from build123d import *

# Parameters (mm, degrees)
CUT_EXTRUDE_12_DEPTH      = 102.948516419
CUT_EXTRUDE_12_DEPTH_BACK = 102.948516419
CUT_EXTRUDE_START         = 61
CUT_EXTRUDE_5_R0_25_DEPTH = 31


with BuildPart() as part:
    # Эскиз1 → Revolve 289 (revolve)
    with BuildSketch(Plane.XY, mode=Mode.PRIVATE) as revolve_289_sk:
        with BuildLine():
            Line((0, 32.5), (37, 32.5))
            Line((37, 32.5), (64.745695, 25.068113))
            ThreePointArc((64.745695, 25.068113), (65.002224223, 25.017098236), (65.263217049, 24.999995817))
            Line((65.263217049, 24.999995817), (69.749999449, 24.999995817))
            Line((69.749999449, 24.999995817), (70.749999449, 23.999995817))
            Line((70.749999449, 23.999995817), (70.749999449, 19.499995817))
            Line((70.749999449, 19.499995817), (79.25, 19.499995817))
            Line((79.25, 19.499995817), (79.25, 24))
            Line((79.25, 24), (80.25, 25))
            Line((80.25, 25), (88, 25))
            Line((88, 25), (91, 22))
            Line((91, 22), (91, 11))
            Line((91, 11), (90, 10))
            Line((90, 10), (61, 10))
            Line((61, 10), (61, 19))
            ThreePointArc((61, 19), (60.707106781, 19.707106781), (60, 20))
            Line((60, 20), (25, 20))
            Line((25, 20), (25, 27.1))
            ThreePointArc((25, 27.1), (24.882842712, 27.382842712), (24.6, 27.5))
            Line((24.6, 27.5), (0, 27.5))
            Line((0, 27.5), (0, 32.5))
        make_face()
    revolve(revolve_289_sk.sketch.rotate(Axis((0, 0, 0), (1, 0, 0)), 90), axis=Axis((0, 0, 0), (1, 0, 0)))

    # Эскиз2 → Наклон торца 12 градусов (cut, two sides: drawn at the far end of the back side and taken through both)
    with BuildSketch(Plane(origin=(0, 0, 0), x_dir=(1, 0, 0), z_dir=(0, 1, 0)).offset(-CUT_EXTRUDE_12_DEPTH_BACK)):
        Polygon((-25, 50), (15.30407244, 50), (-5.951583727, -50), (-25, -50), align=None)
    extrude(amount=CUT_EXTRUDE_12_DEPTH + CUT_EXTRUDE_12_DEPTH_BACK, mode=Mode.SUBTRACT)

    # Эскиз3 → Паз 5 R0.25 (cut)
    with BuildSketch(Plane(origin=(0, 0, 0), x_dir=(0, 0, -1), z_dir=(1, 0, 0)).offset(CUT_EXTRUDE_START)):
        with BuildLine():
            Line((0, -2.5), (0, 2.5))
            Line((0, 2.5), (-12.05, 2.5))
            ThreePointArc((-12.05, 2.5), (-12.226776695, 2.426776695), (-12.3, 2.25))
            Line((-12.3, 2.25), (-12.3, -2.25))
            ThreePointArc((-12.3, -2.25), (-12.226776695, -2.426776695), (-12.05, -2.5))
            Line((-12.05, -2.5), (0, -2.5))
        make_face()
    extrude(amount=CUT_EXTRUDE_5_R0_25_DEPTH, mode=Mode.SUBTRACT)

    # Эскиз4 → Cut-Revolve M4 30 -1 (revolve, cut)
    with BuildSketch(Plane(origin=(0, 0, 0), x_dir=(1, 0, 0), z_dir=(0, -0.49999999999999994, 0.8660254037844387)), mode=Mode.PRIVATE) as cut_revolve_m4_30_1_sk:
        Polygon((17, -26), (18.7, -26), (18.7, -29.5), (20.5, -29.5), (20.5, -40), (17, -40), align=None)
    revolve(cut_revolve_m4_30_1_sk.sketch.rotate(Axis((17, -17.320508076, -10), (0, -0.8660254037844387, -0.49999999999999994)), 90), axis=Axis((17, -17.320508076, -10), (0, -0.8660254037844387, -0.49999999999999994)), mode=Mode.SUBTRACT)

    # Эскиз5 → Cut-Revolve M4 30 1 2 (revolve, cut)
    with BuildSketch(Plane(origin=(0, 0, 0), x_dir=(1, 0, 0), z_dir=(0, -0.49999999999999994, 0.8660254037844387)), mode=Mode.PRIVATE) as cut_revolve_m4_30_1_2_sk:
        Polygon((17, 26), (18.7, 26), (18.7, 29.5), (20.5, 29.5), (20.5, 40), (17, 40), align=None)
    revolve(cut_revolve_m4_30_1_2_sk.sketch.rotate(Axis((17, 17.320508076, 10), (0, 0.8660254037844387, 0.49999999999999994)), 90), axis=Axis((17, 17.320508076, 10), (0, 0.8660254037844387, 0.49999999999999994)), mode=Mode.SUBTRACT)

    # Эскиз6 → Cut-Revolve M4 150 -1 (revolve, cut)
    with BuildSketch(Plane(origin=(0, 0, 0), x_dir=(1, 0, 0), z_dir=(0, -0.49999999999999994, -0.8660254037844387)), mode=Mode.PRIVATE) as cut_revolve_m4_150_1_sk:
        Polygon((17, -26), (18.7, -26), (18.7, -29.5), (20.5, -29.5), (20.5, -40), (17, -40), align=None)
    revolve(cut_revolve_m4_150_1_sk.sketch.rotate(Axis((17, 17.320508076, -10), (0, 0.8660254037844387, -0.49999999999999994)), 90), axis=Axis((17, 17.320508076, -10), (0, 0.8660254037844387, -0.49999999999999994)), mode=Mode.SUBTRACT)

    # Эскиз7 → Cut-Revolve M4 150 1 2 (revolve, cut)
    with BuildSketch(Plane(origin=(0, 0, 0), x_dir=(1, 0, 0), z_dir=(0, -0.49999999999999994, -0.8660254037844387)), mode=Mode.PRIVATE) as cut_revolve_m4_150_1_2_sk:
        Polygon((17, 26), (18.7, 26), (18.7, 29.5), (20.5, 29.5), (20.5, 40), (17, 40), align=None)
    revolve(cut_revolve_m4_150_1_2_sk.sketch.rotate(Axis((17, -17.320508076, 10), (0, -0.8660254037844387, 0.49999999999999994)), 90), axis=Axis((17, -17.320508076, 10), (0, -0.8660254037844387, 0.49999999999999994)), mode=Mode.SUBTRACT)

    # Эскиз8 → Радиальное отверстие 3.6 цековка 7 (revolve, cut)
    with BuildSketch(Plane(origin=(0, 0, 0), x_dir=(1, 0, 0), z_dir=(0, 1, 0)), mode=Mode.PRIVATE) as cut_revolve_3_6_7_sk:
        Polygon((78, -8), (79.8, -8), (79.8, -15), (81.5, -15), (81.5, -35), (78, -35), align=None)
    revolve(cut_revolve_3_6_7_sk.sketch.rotate(Axis((78, 0, 0), (0, 0, 1)), 180), axis=Axis((78, 0, 0), (0, 0, 1)), mode=Mode.SUBTRACT)


solid = part.part
Geometry: final body of the model. Coordinates: model frame, mm. A direction names the side the tool comes from. Round coordinates to 2 decimals unless told otherwise and drop trailing zeros. Loops run counter-clockwise (first coordinate to the right, second up) from the corner with the lowest first, then second, coordinate; pieces in that order, holes last. Notation, with made-up numbers: M -29,-11 L 25,-11 A30 ccw 25,13 Z; hole C -24,24 d7. An arc over 180 degrees is marked long. One line per question, with ' | ' between items.
(1) Cut plane C-C on x = 49. Return the cut outline in (y, z), plus the area to 3 significant figures.
Check result:
outline: C 0,0 d58.57; hole C 0,0 d40 | area: 1,440 mm2
(2) Cut plane A-A on x = 72.5. Return the cut outline in (y, z).
Check result:
outline: C 0,0 d39; hole M -2.5,9.68 A10 ccw long 2.5,9.68 L 2.5,12.05 A0.25 ccw 2.25,12.3 L -2.25,12.3 A0.25 ccw -2.5,12.05 Z
(3) Contact query for flat-ended pins moving along their axis: P1, Ø8, axis at y = -12, z = -13, coming from the -X side; P2, Ø0.7, axis at x = 80.5, z = 11, coming from the +Y side; P3, Ø1.2, axis at x = 70.5, z = 11, coming from the -Y side; P4, Ø16, axis at y = 0, z = 0, coming from the +X side. Output: stop coordinate, or through.
Check result:
P1: stops at x = 25 | P2: stops at y = 22.62 | P3: stops at y = -22.34 | P4: passes through
(4) Cut plane B-B on y = 0. Give the number of separate pieces and of enclosed holes in the cut face, plus the area to 3 significant figures.
Check result:
separate pieces: 3 | enclosed holes: 0 | area: 1,620 mm2
(5) Access query for faces 5 (the cylindrical face through (67.538, 24.406, -5.42)), 6 (the cylindrical face through (42.26, -0.88, -19.98)), 7 (the cylindrical face through (81.497, -0.154, 18.959)). Directions: +Z, -Z, +X, -X, +Y, -Y. A direction counts if a zero-diameter tool reaches every point of the face in a straight line with its end or side. Return the directions, or none.
Check result:
face 5: +X | face 6: -X | face 7: +Z
(6) Material intervals for line 1 along X through (y, z) = (-16.5, 13); line 2 along Y through (x, z) = (69, 0); line 3 along X through (y, z) = (13, 19), sorted ascending. Write a range as from..to.
Check result:
line 1: x = 25..70.75, 79.25..91 | line 2: y = -25..-10, 10..25 | line 3: x = 25..70.75, 79.25..89.98
(7) Pull-direction query (Y, two-part tool) for faces 1 (the cylindrical face through (15.57, -25.13, -13.45)), 2 (the flat face through (0, 0, 28)), 3 (the flat face through (77, -2, 15)), 4 (the conical face through (79.42, -1.03, -24.15)); classes: +Y half, -Y half, draft (parallel to the pull), parting line (faces both ways), or undercut.
Check result:
face 1: undercut | face 2: draft | face 3: undercut | face 4: parting line
